Check sheet for the modelled part. Datum: model origin and axes. Units: mm. A direction names the side the tool comes from. Round coordinates to 2 decimals unless told otherwise and drop trailing zeros. Write each loop counter-clockwise with the first axis right and the second up, starting at its lowest first coordinate (ties: lowest second). Pieces come first, ordered by that corner, then holes. Notation, with made-up numbers: M 61,11 L 107,11 A20 ccw 107,21 Z; hole C 15.25,49.25 d1. An arc over 180 degrees is marked long. Answer in a Markdown table with one row per item.
```python
from build123d import *

# Parameters (mm, degrees)
EXTRUDE_1_DEPTH                    = 2.55
CUT_EXTRUDE_1_DEPTH                = 9.2
EXTRUDE_2_DEPTH                    = 3.8
SKETCH_4_W                         = 5.63
SKETCH_4_H                         = 1
CUT_EXTRUDE_2_DEPTH                = 3.8
CUT_EXTRUDE_3_REACH                = 16.445
CHAMFER_1_SIZE                     = 0.5
EXTRUDE_START                      = -3.6
SKETCH_6_W                         = 0.64
SKETCH_6_H                         = 0.64
EXTRUDE_3_DEPTH                    = 11.7
CHAMFER_2_SIZE                     = 0.2
PATTERN_LINEAR_1_COUNT             = 3
PATTERN_LINEAR_1_PITCH             = 2.54
CHAMFER_2_OF_PATTERN_LINEAR_1_SIZE = 0.2


with BuildPart() as part:
    # Эскиз1 → Бобышка-Вытянуть1 (new, symmetric)
    with BuildSketch(Plane(origin=(0, 0, 0), x_dir=(1, 0, 0), z_dir=(0, 1, 0))):
        Polygon((-3.685, -0.3), (3.685, -0.3), (3.685, 0), (4.385, 0), (4.385, -0.3), (5.085, -0.3), (5.085, -11.8), (-5.085, -11.8), (-5.085, -0.3), (-4.385, -0.3), (-4.385, 0), (-3.685, 0), align=None)
    extrude(amount=EXTRUDE_1_DEPTH, both=True)

    # Эскиз2 → Вырез-Вытянуть1 (cut)
    with BuildSketch(Plane.XY.offset(11.8)):
        Polygon((-4.085, 1.55), (-4.085, -1.55), (0.67, -1.55), (0.67, -2.55), (1.87, -2.55), (1.87, -1.55), (4.085, -1.55), (4.085, 1.55), (1.5, 1.55), (1.5, 2.55), (-1.5, 2.55), (-1.5, 1.55), align=None)
    extrude(amount=-CUT_EXTRUDE_1_DEPTH, mode=Mode.SUBTRACT)

    # Эскиз3 → Бобышка-Вытянуть2 (add)
    with BuildSketch(Plane.XY.offset(11.8)):
        Polygon((-3.815, 2.55), (-3.815, 4.05), (3.815, 4.05), (3.815, 2.55), (2.815, 2.55), (2.815, 3.05), (-2.815, 3.05), (-2.815, 2.55), align=None)
    extrude(amount=-EXTRUDE_2_DEPTH)

    # Эскиз4 → Вырез-Вытянуть2 (cut)
    with BuildSketch(Plane.XY.offset(11.8)):
        with Locations((0, 2.05)):
            Rectangle(SKETCH_4_W, SKETCH_4_H)
    extrude(amount=-CUT_EXTRUDE_2_DEPTH, mode=Mode.SUBTRACT)

    # Эскиз5 → Вырез-Вытянуть3 (cut, up to next)
    with BuildSketch(Plane(origin=(0, 4.05, 0), x_dir=(1, 0, 0), z_dir=(0, 1, 0)), mode=Mode.PRIVATE) as cut_extrude_3_sk1:
        with BuildLine():
            Line((2.815, -8), (2.815, -9.8))
            ThreePointArc((2.815, -9.8), (2.668553391, -10.153553391), (2.315, -10.3))
            Line((2.315, -10.3), (-2.315, -10.3))
            ThreePointArc((-2.315, -10.3), (-2.668553391, -10.153553391), (-2.815, -9.8))
            Line((-2.815, -9.8), (-2.815, -8))
            Line((-2.815, -8), (2.815, -8))
        make_face()
    cut_extrude_3_tool1 = extrude(cut_extrude_3_sk1.sketch, amount=-CUT_EXTRUDE_3_REACH, mode=Mode.PRIVATE) & part.part
    add(cut_extrude_3_tool1.solids().sort_by_distance((0, 4.05, 9.141324))[0], mode=Mode.SUBTRACT)

    # Фаска1
    chamfer_1_edges = [part.edges().sort_by_distance(p)[0] for p in [
        (-2.1575, 1.55, 8),
        (-4.085, 0, 11.8),
        (-1.7075, -1.55, 11.8),
        (2.9775, -1.55, 11.8),
        (4.085, 0, 11.8),
        (3.45, 1.55, 11.8),
        (-2.815, 2.3, 11.8),
        (0, 3.05, 11.8),
        (2.815, 2.3, 11.8),
        (2.1575, 1.55, 8),
        (-3.45, 1.55, 11.8),
    ]]
    chamfer(chamfer_1_edges, length=CHAMFER_1_SIZE)

    # Эскиз6 → Бобышка-Вытянуть3 (add)
    with BuildSketch(Plane.XY.offset(0.3).offset(EXTRUDE_START)):
        with Locations((2.54, 0)):
            Rectangle(SKETCH_6_W, SKETCH_6_H)
    extrude_3 = extrude(amount=EXTRUDE_3_DEPTH)

    # Фаска2
    chamfer_2_edges = [part.edges().sort_by_distance(p)[0] for p in [
        (2.54, 0.32, 8.4),
        (2.86, 0, 8.4),
        (2.54, -0.32, 8.4),
        (2.22, 0, 8.4),
        (2.22, 0, -3.3),
        (2.54, 0.32, -3.3),
        (2.86, 0, -3.3),
        (2.54, -0.32, -3.3),
    ]]
    chamfer(chamfer_2_edges, length=CHAMFER_2_SIZE)

    # Линейный массив1: Бобышка-Вытянуть3 ×3
    with Locations(*[(-i * PATTERN_LINEAR_1_PITCH, 0, 0) for i in range(1, PATTERN_LINEAR_1_COUNT)]):
        add(extrude_3)

    # Фаска2 of Линейный массив1
    chamfer_2_of_pattern_linear_1_edges = [part.edges().sort_by_distance(p)[0] for p in [
        (0, 0.32, 8.4),
        (0.32, 0, 8.4),
        (0, -0.32, 8.4),
        (-0.32, 0, 8.4),
        (-0.32, 0, -3.3),
        (0, 0.32, -3.3),
        (0.32, 0, -3.3),
        (0, -0.32, -3.3),
        (-2.54, 0.32, 8.4),
        (-2.22, 0, 8.4),
        (-2.54, -0.32, 8.4),
        (-2.86, 0, 8.4),
        (-2.86, 0, -3.3),
        (-2.54, 0.32, -3.3),
        (-2.22, 0, -3.3),
        (-2.54, -0.32, -3.3),
    ]]
    chamfer(chamfer_2_of_pattern_linear_1_edges, length=CHAMFER_2_OF_PATTERN_LINEAR_1_SIZE)


solid = part.part
```
1. Go/stop test with flat-tipped pins: pin 1 (1.1 mm diameter, centred on x = -3, y = 3, fed in from -Z); pin 2 (6 mm diameter, centred on x = 4, z = 0.5, fed in from +Y); pin 3 (0.8 mm diameter, centred on y = 3.5, z = 9.5, fed in from -X) (3 decimals). Record where each tip stops, or that it passes through.
Found:
| item | result |
|---|---|
| pin 1 | stops at z = 0.3 |
| pin 2 | stops at y = 2.55 |
| pin 3 | stops at x = -3.815 |
2. Section check B-B, the plane z = -1.75. Record the cut outline in (x, y).
Found:
| item | result |
|---|---|
| outline | M -2.86,-0.32 L -2.22,-0.32 L -2.22,0.32 L -2.86,0.32 Z; M -0.32,-0.32 L 0.32,-0.32 L 0.32,0.32 L -0.32,0.32 Z; M 2.22,-0.32 L 2.86,-0.32 L 2.86,0.32 L 2.22,0.32 Z |
3. Section check A-A, the plane x = -1. Record the cut outline in (y, z).
Found:
| item | result |
|---|---|
| outline | M -2.55,0.3 L 2.55,0.3 L 2.55,2.6 L -1.55,2.6 L -1.55,11.3 L -2.05,11.8 L -2.55,11.8 Z; M 3.05,10.3 L 4.05,10.3 L 4.05,11.8 L 3.55,11.8 L 3.05,11.3 Z |
4. Draft check along Y on faces 6 (the face through (3.815, 3, 10)), 7 (the face through (0, 4.05, 11)), 8 (the face through (2.815, 3, 9)). Enter one of: +Y half, -Y half, draft (parallel to the pull), parting line (faces both ways), or undercut.
Found:
| item | result |
|---|---|
| face 6 | draft |
| face 7 | +Y half |
| face 8 | undercut |
5. Access from +Z, -Z, +X, -X, +Y, -Y to the whole of each face (thin tool, end or side, straight path). Record for faces 1 (the face through (0.67, -2, 7)), 2 (the face through (-3, 1.55, 6)), 3 (the face through (3, 3, 8)), 4 (the face through (1.5, 2, 5)), 5 (the face through (0, 3.05, 11)).
Found:
| item | result |
|---|---|
| face 1 | +Z, -Y |
| face 2 | +Z |
| face 3 | -Z, +X, -X, +Y |
| face 4 | +Z, +Y, -Y |
| face 5 | +Z, -Z |
6. Section check C-C, the plane z = 4. Record the cut outline in (x, y) (3 decimals), and give its area (3 significant figures).
Found:
| item | result |
|---|---|
| outline | M -5.085,-2.55 L 0.67,-2.55 L 0.67,-1.55 L -4.085,-1.55 L -4.085,1.55 L -1.5,1.55 L -1.5,2.55 L -5.085,2.55 Z; M -2.86,-0.32 L -2.22,-0.32 L -2.22,0.32 L -2.86,0.32 Z; M -0.32,-0.32 L 0.32,-0.32 L 0.32,0.32 L -0.32,0.32 Z; M 1.5,1.55 L 4.085,1.55 L 4.085,-1.55 L 1.87,-1.55 L 1.87,-2.55 L 5.085,-2.55 L 5.085,2.55 L 1.5,2.55 Z; M 2.22,-0.32 L 2.86,-0.32 L 2.86,0.32 L 2.22,0.32 Z |
| area | 23.6 mm2 |
7. Section check D-D, the plane y = 0.75. Record the cut outline in (x, z) (3 decimals), and give its area (3 significant figures).
Found:
| item | result |
|---|---|
| outline | M -5.085,0.3 L -4.385,0.3 L -4.385,0 L -3.685,0 L -3.685,0.3 L 3.685,0.3 L 3.685,0 L 4.385,0 L 4.385,0.3 L 5.085,0.3 L 5.085,11.8 L 4.585,11.8 L 4.085,11.3 L 4.085,2.6 L -4.085,2.6 L -4.085,11.3 L -4.585,11.8 L -5.085,11.8 Z |
| area | 42.0 mm2 |
8. Scan lines: L1, parallel to X at y = 2.25, z = 10.75 (3 decimals); L2, parallel to X at y = -0.75, z = 5.5 (3 decimals); L3, parallel to Y at x = -3.25, z = 11.25. Record each from-to range of solid material in increasing order.
Found:
| item | result |
|---|---|
| L1 | x = -5.085 to -2.815, 2.815 to 5.085 |
| L2 | x = -5.085 to -4.085, 4.085 to 5.085 |
| L3 | y = -2.55 to -1.55, 1.55 to 4.05 |
